from build123d import *

# Parameters (mm, degrees)
BOSS_EXTRUDE1_DEPTH = 152.4
FILLET1_R           = 25.4


with BuildPart() as part:
    # Sketch1 → Boss-Extrude1 (new body)
    with BuildSketch(Plane(origin=(0, 0, 0), x_dir=(1, 0, 0), z_dir=(0, 1, 0))):
        Polygon((228.6, 0), (0, 0), (0, -977.9), (854.075, -977.9), (854.075, 0), (625.475, 0), (625.475, -76.2), (777.875, -76.2), (777.875, -901.7), (76.2, -901.7), (76.2, -76.2), (228.6, -76.2), align=None)
    extrude(amount=BOSS_EXTRUDE1_DEPTH)

    # Fillet1
    fillet1_edges = [part.edges().sort_by_distance(p)[0] for p in [
        (0, 152.4, 488.95),
        (427.0375, 152.4, 977.9),
        (739.775, 0, 0),
        (854.075, 0, 488.95),
        (427.0375, 0, 977.9),
        (0, 0, 488.95),
        (114.3, 0, 0),
        (854.075, 152.4, 488.95),
        (739.775, 152.4, 0),
        (625.475, 76.2, 0),
        (854.075, 76.2, 0),
        (854.075, 76.2, 977.9),
        (0, 76.2, 977.9),
        (0, 76.2, 0),
        (228.6, 76.2, 0),
        (114.3, 152.4, 0),
    ]]
    fillet(fillet1_edges, radius=FILLET1_R)


solid = part.part
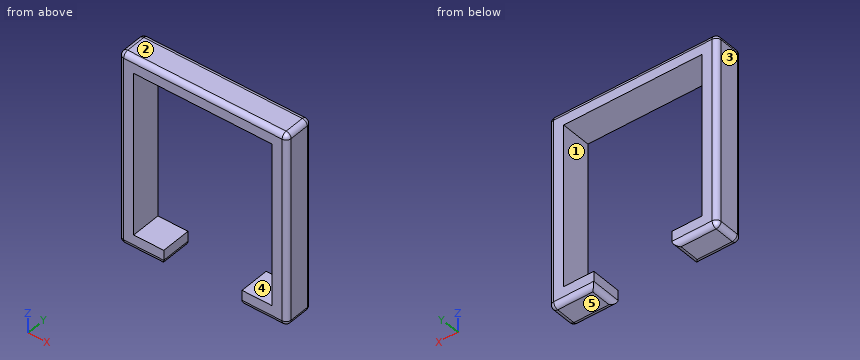
Verification items for the finished model (mm, model axes). Face numbers are marked on the shaded views. A direction names the side the tool comes from. Give positions to 0.01 mm unless a question says otherwise; leave off trailing zeros. Loops run counter-clockwise (first coordinate to the right, second up) from the corner with the lowest first, then second, coordinate; pieces in that order, holes last.
1. Material ranges on probe 1 along X at (y, z) = (105.5, 846) (3 decimals); probe 2 along X at (y, z) = (105, 74) (3 decimals); probe 3 along Z at (x, y) = (182, 88), recorded low to high.
Derived:
probe 1: x = 0 to 76.2, 777.875 to 854.075
probe 2: x = 0 to 228.6, 625.475 to 854.075
probe 3: z = 0 to 76.2, 901.7 to 977.9
2. Cross-section at C-C on z = 358.5. Record the cut outline in (x, y) (3 decimals), and give its area (3 significant figures).
Derived:
outline: (0, 25.4) arc R25.4 ccw to (25.4, 0) - (76.2, 0) - (76.2, 152.4) - (25.4, 152.4) arc R25.4 ccw to (0, 127) - close; (777.875, 0) - (828.675, 0) arc R25.4 ccw to (854.075, 25.4) - (854.075, 127) arc R25.4 ccw to (828.675, 152.4) - (777.875, 152.4) - close
area: 22,700 mm2
3. Tool access check on the marked faces 1 and 2. Record the directions out of +Z, -Z, +X, -X, +Y, -Y that give a thin tool (end or side, any length) a straight path to the whole face; none if there is none.
Derived:
face 1: +Y, -Y
face 2: +Z, +X, -X, +Y, -Y
4. Cross-section at B-B on y = 115.5. Record the cut outline in (x, z) (3 decimals).
Derived:
outline: (0, 25.4) arc R25.4 ccw to (25.4, 0) - (203.2, 0) arc R25.4 ccw to (228.6, 25.4) - (228.6, 76.2) - (76.2, 76.2) - (76.2, 901.7) - (777.875, 901.7) - (777.875, 76.2) - (625.475, 76.2) - (625.475, 25.4) arc R25.4 ccw to (650.875, 0) - (828.675, 0) arc R25.4 ccw to (854.075, 25.4) - (854.075, 952.5) arc R25.4 ccw to (828.675, 977.9) - (25.4, 977.9) arc R25.4 ccw to (0, 952.5) - close
5. Go/stop test with flat-tipped pins: P1, Ø2, axis at x = 593.5, y = 79, coming from the -Z side; P2, Ø3, axis at x = 296, y = 131.5, coming from the +Z side. Record where each tip stops, or that it passes through.
Derived:
P1: stops at z = 901.7
P2: stops at z = 977.72
6. Cross-section at D-D on x = 342.5. Record the cut outline in (y, z).
Derived:
outline: (0, 901.7) - (152.4, 901.7) - (152.4, 952.5) arc R25.4 ccw to (127, 977.9) - (25.4, 977.9) arc R25.4 ccw to (0, 952.5) - close
7. Cross-section at A-A on x = 709. Record the cut outline in (y, z), and give its area (3 significant figures).
Derived:
outline: (0, 25.4) arc R25.4 ccw to (25.4, 0) - (127, 0) arc R25.4 ccw to (152.4, 25.4) - (152.4, 76.2) - (0, 76.2) - close; (0, 901.7) - (152.4, 901.7) - (152.4, 952.5) arc R25.4 ccw to (127, 977.9) - (25.4, 977.9) arc R25.4 ccw to (0, 952.5) - close
area: 22,700 mm2
8. Release check for a two-part mould opening along X. For the marked faces 3, 4 and 5 record: +X half, -X half, draft (parallel to the pull), parting line (faces both ways), or undercut.
Derived:
face 3: -X half
face 4: undercut
face 5: draft
